Part model, mm, in its own coordinate system. Face numbers are marked on the shaded views. Give positions to 0.01 mm unless a question says otherwise; leave off trailing zeros. Order: outer loops, then holes, each group sorted by start corner. A loop starts at its lowest first (then second) coordinate and runs counter-clockwise, first axis right, second up. Notation, with made-up numbers: M 59,-37 L 114,-37 A25 cw 114,2 Z; hole C -22.75,73 d6. An arc over 180 degrees is marked long. Return JSON: item names as keys, results as strings.
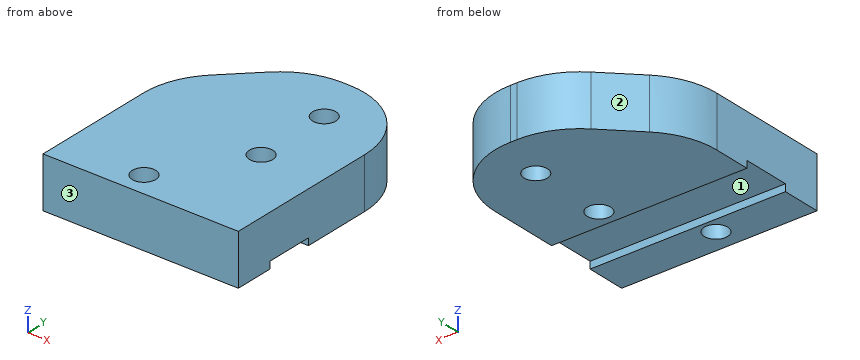
from build123d import *

# Parameters (mm, degrees)
F0_W     = 25
F0_H     = 30
F1_DEPTH = 6.5
F2_R     = 1.5
F3_DEPTH = 6.501
F4_W     = 25
F4_H     = 6.1
F5_DEPTH = 0.9
F6_SIZE  = 10
F7_R     = 10


with BuildPart() as f1:
    # F0 (on Top) → F1 (new body)
    with BuildSketch(Plane.XY):
        Rectangle(F0_W, F0_H)
    extrude(amount=F1_DEPTH)

    # F2 (on face) → F3 (cut, through all)
    with BuildSketch(Plane.XY.offset(6.5)):
        with Locations((-2, -12)):
            Circle(F2_R)
        with Locations((4.5, -1.5)):
            Circle(F2_R)
        with Locations((4.5, 8.5)):
            Circle(F2_R)
    extrude(amount=-F3_DEPTH, mode=Mode.SUBTRACT)

    # F4 (on face) → F5 (cut)
    with BuildSketch(Plane(origin=(0, 0, 0), x_dir=(1, 0, 0), z_dir=(0, 0, -1))):
        with Locations((0, 6.95)):
            Rectangle(F4_W, F4_H)
    extrude(amount=-F5_DEPTH, mode=Mode.SUBTRACT)

    # F6
    f6_edges = [f1.edges().sort_by_distance(p)[0] for p in [
        (-12.5, 15, 3.25),
    ]]
    chamfer(f6_edges, length=F6_SIZE)

    # F7
    f7_edges = [f1.edges().sort_by_distance(p)[0] for p in [
        (-12.5, 5, 3.25),
        (-2.5, 15, 3.25),
        (12.5, 15, 3.25),
    ]]
    fillet(f7_edges, radius=F7_R)


solid = f1.part
Q1. Band-saw the part on D-D (x = -6). Give the cut face in (y, z), then the cut area to 3 significant figures.
Established:
{"outline": "M -15,0 L -10,0 L -10,0.9 L -3.9,0.9 L -3.9,0 L 11.5,0 L 11.5,6.5 L -15,6.5 Z", "area": "167 mm²"}
Q2. Band-saw the part on C-C (x = 4.5). Give the cut face in (y, z), then the cut area to 3 significant figures.
Established:
{"outline": "M -15,0 L -10,0 L -10,0.9 L -3.9,0.9 L -3.9,0 L -3,0 L -3,6.5 L -15,6.5 Z; M 0,0 L 7,0 L 7,6.5 L 0,6.5 Z; M 10,0 L 14.8,0 L 14.8,6.5 L 10,6.5 Z", "area": "149 mm²"}
Q3. Band-saw the part on B-B (y = -12). Give the cut face in (x, z), then the cut area to 3 significant figures.
Established:
{"outline": "M -12.5,0 L -3.5,0 L -3.5,6.5 L -12.5,6.5 Z; M -0.5,0 L 12.5,0 L 12.5,6.5 L -0.5,6.5 Z", "area": "143 mm²"}
Q4. Two-plate mould, pull along Y, no slides. Class the marked faces 1, 2 and 3: +Y half, -Y half, draft (parallel to the pull), parting line (faces both ways), or undercut.
Established:
{"face 1": "undercut", "face 2": "+Y half", "face 3": "-Y half"}
Q5. Band-saw the part on A-A (z = 3). Give the cut face in (x, y), then the cut area to 3 significant figures.
Established:
{"outline": "M -12.5,-15 L 12.5,-15 L 12.5,5 A10 ccw 2.5,15 L 1.64,15 A10 ccw -5.43,12.07 L -9.57,7.93 A10 ccw -12.5,0.86 Z; hole C -2,-12 d3; hole C 4.5,-1.5 d3; hole C 4.5,8.5 d3", "area": "653 mm²"}
Q6. Pin check, flat tips, straight feed: pin 1 (1 mm diameter, centred on x = -6, z = 0.5, fed in from +Y); pin 2 (1.8 mm diameter, centred on x = -2.5, y = -6.5, fed in from -Z); pin 3 (5 mm diameter, centred on x = -2, y = -12, fed in from +Z). Stop position of each tip, or through.
Established:
{"pin 1": "stops at y = 12", "pin 2": "stops at z = 0.9", "pin 3": "stops at z = 6.5"}
Q7. Probe line 1 along Y through (x, z) = (4.5, 1.75); line 2 along Y through (x, z) = (3.75, 2.5); line 3 along Z through (x, y) = (1, -7). List the from-to ranges inside material, lowest first.
Established:
{"line 1": "y = -15 to -3, 0 to 7, 10 to 14.8", "line 2": "y = -15 to -2.8, -0.2 to 7.2, 9.8 to 14.92", "line 3": "z = 0.9 to 6.5"}
